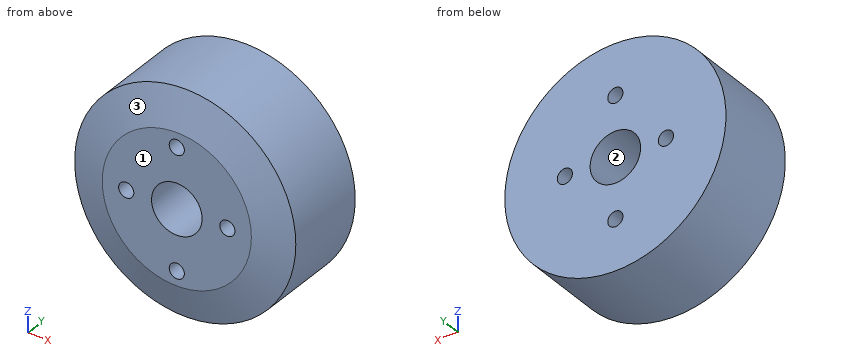
```python
from build123d import *

# Parameters (mm, degrees)
F0_R     = 17.5
F0_R_2   = 4
F1_DEPTH = 15.3
F2_SIZE2 = 1.9
F2_SIZE  = 5.7
F4_D     = 2.4


with BuildPart() as f1:
    # F0 (on Front) → F1 (new body)
    with BuildSketch(Plane.XZ):
        Circle(F0_R)
        Circle(F0_R_2, mode=Mode.SUBTRACT)
    extrude(amount=F1_DEPTH)

    # F2
    f2_edges = [f1.edges().sort_by_distance(p)[0] for p in [
        (-17.5, -15.3, 0),
    ]]
    f2_side = f1.faces().sort_by_distance((-17.005025, -15.3, 0))[0]
    chamfer(f2_edges, length=F2_SIZE, length2=F2_SIZE2, reference=f2_side)

    # F4 (through all)
    with Locations(Plane.XZ.offset(15.3)):
        with Locations((0, 9.5), (-8, 0), (0, -9.5), (8, 0)):
            Hole(F4_D / 2)


solid = f1.part
```
Input: part model. Units: mm. Frame: model coordinates. Face numbers are marked on the shaded views. Give positions to 0.01 mm unless a question says otherwise; leave off trailing zeros. Loops run counter-clockwise (first coordinate to the right, second up) from the corner with the lowest first, then second, coordinate; pieces in that order, holes last. Notation, with made-up numbers: (-19, -2.75) -> (24, -2.75) arc R12 cw to (24, 17.25) -> close; hole circle Ø11 at (24, 8). An arc over 180 degrees is marked (long way). Use a Markdown table: item, result.
Q1. Pull-direction query (Z, two-part tool) for the marked faces 1, 2 and 3; classes: pulls with the +Z half, pulls with the -Z half, needs draft (parallel to the pull), parting line crosses it, or undercut.
Entries:
| item | result |
|---|---|
| face 1 | needs draft |
| face 2 | undercut |
| face 3 | parting line crosses it |
Q2. Ray query, probe 1 along Z at (x, y) = (0, -10); probe 2 along Z at (x, y) = (1, -9.5); probe 3 along Z at (x, y) = (-8, -6.75). Return the intervals inside material, ascending. Write a range as from..to.
Entries:
| item | result |
|---|---|
| probe 1 | z = -17.5..-10.7, -8.3..-4, 4..8.3, 10.7..17.5 |
| probe 2 | z = -17.47..-10.16, -8.84..-3.87, 3.87..8.84, 10.16..17.47 |
| probe 3 | z = -15.56..-1.2, 1.2..15.56 |
Q3. Section query C-C, the plane y = -9. Return the cut outline in (x, z).
Entries:
| item | result |
|---|---|
| outline | circle Ø35 at (0, 0); hole circle Ø2.4 at (-8, 0); hole circle Ø8 at (0, 0); hole circle Ø2.4 at (0, -9.5); hole circle Ø2.4 at (0, 9.5); hole circle Ø2.4 at (8, 0) |
Q4. First-contact query: P1, Ø6, axis at x = 1, z = -4, coming from the +Y side; P2, Ø4, axis at x = -6.5, y = -2, coming from the +Z side; P3, Ø1.4, axis at x = 0, z = -9.5, coming from the +Y side; P4, Ø2, axis at y = -12, z = -14, coming from the +X side. Flat tips, straight axial feed; report the tip coordinate or a pass-through.
Entries:
| item | result |
|---|---|
| P1 | stops at y = 0 |
| P2 | stops at z = 16.91 |
| P3 | passes through |
| P4 | stops at x = 11.72 |
Q5. Section query B-B, the plane x = 0. Return the cut outline in (y, z), plus the area to 3 significant figures.
Entries:
| item | result |
|---|---|
| outline | (-15.3, -11.8) -> (-13.4, -17.5) -> (0, -17.5) -> (0, -10.7) -> (-15.3, -10.7) -> close; (-15.3, -8.3) -> (0, -8.3) -> (0, -4) -> (-15.3, -4) -> close; (-15.3, 4) -> (0, 4) -> (0, 8.3) -> (-15.3, 8.3) -> close; (-15.3, 10.7) -> (0, 10.7) -> (0, 17.5) -> (-13.4, 17.5) -> (-15.3, 11.8) -> close |
| area | 329 mm² |
Q6. Section query A-A, the plane z = 0. Return the cut outline in (x, y), plus the area to 3 significant figures.
Entries:
| item | result |
|---|---|
| outline | (-17.5, -13.4) -> (-11.8, -15.3) -> (-9.2, -15.3) -> (-9.2, 0) -> (-17.5, 0) -> close; (-6.8, -15.3) -> (-4, -15.3) -> (-4, 0) -> (-6.8, 0) -> close; (4, -15.3) -> (6.8, -15.3) -> (6.8, 0) -> (4, 0) -> close; (9.2, -15.3) -> (11.8, -15.3) -> (17.5, -13.4) -> (17.5, 0) -> (9.2, 0) -> close |
| area | 329 mm² |
